Source: CAD feature listing. Evaluate the final solid. Frame: model axes, mm. Give positions to 0.01 mm unless a question says otherwise; leave off trailing zeros. Loops run counter-clockwise (first coordinate to the right, second up) from the corner with the lowest first, then second, coordinate; pieces in that order, holes last. Notation, with made-up numbers: (-15.75, 56) -> (20.25, 56) arc R25 ccw to (20.25, 68) -> close; hole circle Ø10 at (48, 8). An arc over 180 degrees is marked (long way). Return JSON: item names as keys, results as strings. Group by question number.
(1) Pin query (flat end, axial travel): pin 1 (2 mm diameter, centred on x = 8.5, z = 3.5, fed in from +Y). Return the tip coordinate at first contact, or that it passes through.
(2) Draft query along X for faces 1 (the face through (-18, 1, 2)), 2 (the face through (-2.246, 4.008, 2.465)), 3 (the face through (-15.746, 3.992, 2.465)). Return one class per face: released by +X, released by -X, zero draft, split by the parting line, or undercut.
(3) Cut plane B-B on y = 3.95. Give the number of separate pieces and of enclosed holes in the cut face, then the cut area to 3 significant figures.
(4) Ray query, line 1 (Y direction, x = 15, z = 4.5); line 2 (X direction, y = 2.65, z = 4.35) (3 decimals); line 3 (Y direction, x = 0.5, z = 3.65). Return the intervals inside material, ascending. Write a range as from..to.
(5) Cut plane A-A on x = 6. Return loops of the section in (y, z).
```python
from build123d import *

# Parameters (mm, degrees)
BOSS_EXTRUDE1_DEPTH = 5


with BuildPart() as part:
    # Sketch2 → Boss-Extrude1 (new body)
    with BuildSketch(Plane.XY):
        with BuildLine():
            Line((-18, 0), (18, 0))
            Line((18, 0), (18, 2.5))
            Line((18, 2.5), (16.947213595, 4.605572809))
            ThreePointArc((16.947213595, 4.605572809), (16.5, 4.881966011), (16.052786405, 4.605572809))
            Line((16.052786405, 4.605572809), (15.447213595, 3.394427191))
            ThreePointArc((15.447213595, 3.394427191), (15, 3.118033989), (14.552786405, 3.394427191))
            Line((14.552786405, 3.394427191), (13.947213595, 4.605572809))
            ThreePointArc((13.947213595, 4.605572809), (13.5, 4.881966011), (13.052786405, 4.605572809))
            Line((13.052786405, 4.605572809), (12.447213595, 3.394427191))
            ThreePointArc((12.447213595, 3.394427191), (12, 3.118033989), (11.552786405, 3.394427191))
            Line((11.552786405, 3.394427191), (10.947213595, 4.605572809))
            ThreePointArc((10.947213595, 4.605572809), (10.5, 4.881966011), (10.052786405, 4.605572809))
            Line((10.052786405, 4.605572809), (9.447213595, 3.394427191))
            ThreePointArc((9.447213595, 3.394427191), (9, 3.118033989), (8.552786405, 3.394427191))
            Line((8.552786405, 3.394427191), (7.947213595, 4.605572809))
            ThreePointArc((7.947213595, 4.605572809), (7.5, 4.881966011), (7.052786405, 4.605572809))
            Line((7.052786405, 4.605572809), (6.447213595, 3.394427191))
            ThreePointArc((6.447213595, 3.394427191), (6, 3.118033989), (5.552786405, 3.394427191))
            Line((5.552786405, 3.394427191), (4.947213595, 4.605572809))
            ThreePointArc((4.947213595, 4.605572809), (4.5, 4.881966011), (4.052786405, 4.605572809))
            Line((4.052786405, 4.605572809), (3.447213595, 3.394427191))
            ThreePointArc((3.447213595, 3.394427191), (3, 3.118033989), (2.552786405, 3.394427191))
            Line((2.552786405, 3.394427191), (1.947213595, 4.605572809))
            ThreePointArc((1.947213595, 4.605572809), (1.5, 4.881966011), (1.052786405, 4.605572809))
            Line((1.052786405, 4.605572809), (0.447213595, 3.394427191))
            ThreePointArc((0.447213595, 3.394427191), (0, 3.118033989), (-0.447213595, 3.394427191))
            Line((-0.447213595, 3.394427191), (-1.052786405, 4.605572809))
            ThreePointArc((-1.052786405, 4.605572809), (-1.5, 4.881966011), (-1.947213595, 4.605572809))
            Line((-1.947213595, 4.605572809), (-2.552786405, 3.394427191))
            ThreePointArc((-2.552786405, 3.394427191), (-3, 3.118033989), (-3.447213595, 3.394427191))
            Line((-3.447213595, 3.394427191), (-4.052786405, 4.605572809))
            ThreePointArc((-4.052786405, 4.605572809), (-4.5, 4.881966011), (-4.947213595, 4.605572809))
            Line((-4.947213595, 4.605572809), (-5.552786405, 3.394427191))
            ThreePointArc((-5.552786405, 3.394427191), (-6, 3.118033989), (-6.447213595, 3.394427191))
            Line((-6.447213595, 3.394427191), (-7.052786405, 4.605572809))
            ThreePointArc((-7.052786405, 4.605572809), (-7.5, 4.881966011), (-7.947213595, 4.605572809))
            Line((-7.947213595, 4.605572809), (-8.552786405, 3.394427191))
            ThreePointArc((-8.552786405, 3.394427191), (-9, 3.118033989), (-9.447213595, 3.394427191))
            Line((-9.447213595, 3.394427191), (-10.052786405, 4.605572809))
            ThreePointArc((-10.052786405, 4.605572809), (-10.5, 4.881966011), (-10.947213595, 4.605572809))
            Line((-10.947213595, 4.605572809), (-11.552786405, 3.394427191))
            ThreePointArc((-11.552786405, 3.394427191), (-12, 3.118033989), (-12.447213595, 3.394427191))
            Line((-12.447213595, 3.394427191), (-13.052786405, 4.605572809))
            ThreePointArc((-13.052786405, 4.605572809), (-13.5, 4.881966011), (-13.947213595, 4.605572809))
            Line((-13.947213595, 4.605572809), (-14.552786405, 3.394427191))
            ThreePointArc((-14.552786405, 3.394427191), (-15, 3.118033989), (-15.447213595, 3.394427191))
            Line((-15.447213595, 3.394427191), (-16.052786405, 4.605572809))
            ThreePointArc((-16.052786405, 4.605572809), (-16.5, 4.881966011), (-16.947213595, 4.605572809))
            Line((-16.947213595, 4.605572809), (-18, 2.5))
            Line((-18, 2.5), (-18, 0))
        make_face()
    extrude(amount=BOSS_EXTRUDE1_DEPTH)


solid = part.part
```
Answers:
{
 "1": {"pin 1": "y = 4.88"},
 "2": {"face 1": "released by -X", "face 2": "undercut", "face 3": "undercut"},
 "3": {"separate pieces": "12", "enclosed holes": "0", "area": "93.0 mm²"},
 "4": {"line 1": "0..3.12", "line 2": "-17.925..17.925", "line 3": "0..3.5"},
 "5": {"outline": "(0, 0) -> (3.12, 0) -> (3.12, 5) -> (0, 5) -> close"}
}
